Geometry: final body of the model. Coordinates: model frame, mm. Give positions to 0.01 mm unless a question says otherwise; leave off trailing zeros. Order: outer loops, then holes, each group sorted by start corner. A loop starts at its lowest first (then second) coordinate and runs counter-clockwise, first axis right, second up. Notation, with made-up numbers: (22, -33.5) -> (26, -33.5) arc R27 ccw to (26, -12.5) -> close; hole circle Ø3 at (56.5, 51.25). An arc over 180 degrees is marked (long way). Write item = value, one per line.
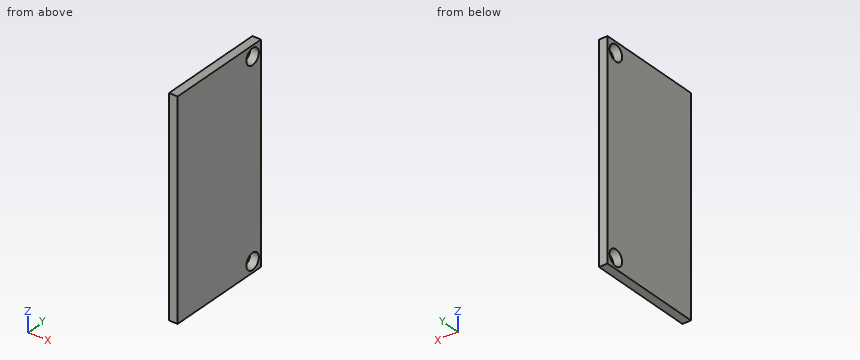
```python
from build123d import *

# Parameters (mm, degrees)
ESQUISSE1_W      = 40
ESQUISSE1_H      = 20
ESQUISSE1_R      = 1.5
EXTRUSION1_DEPTH = 1.6


with BuildPart() as part:
    # Esquisse1 → Extrusion1 (new body)
    with BuildSketch(Plane(origin=(0, 0, 0), x_dir=(0, 0, -1), z_dir=(1, 0, 0))):
        with Locations((0, 10)):
            Rectangle(ESQUISSE1_W, ESQUISSE1_H)
        with Locations((-18, 18)):
            Circle(ESQUISSE1_R, mode=Mode.SUBTRACT)
        with Locations(Location((18, 18, 0), (0, 0, 180))):
            Circle(ESQUISSE1_R, mode=Mode.SUBTRACT)
    extrude(amount=EXTRUSION1_DEPTH)


solid = part.part
```
1) First-contact query: P1, Ø4, axis at y = 10, z = 12.5, coming from the -X side; P2, Ø2.5, axis at y = 18, z = 18, coming from the +X side. Flat tips, straight axial feed; report the tip coordinate or a pass-through.
Check sheet entries:
P1 = 0
P2 = through
2) Section query C-C (x = 1). Output: boundary loops of the cut face in (y, z).
Check sheet entries:
outline = (0, -20) -> (20, -20) -> (20, 20) -> (0, 20) -> close; hole circle Ø3 at (18, -18); hole circle Ø3 at (18, 18)
3) Section query B-B (y = 18). Output: boundary loops of the cut face in (x, z), plus the area to 3 significant figures.
Check sheet entries:
outline = (0, -20) -> (1.6, -20) -> (1.6, -19.5) -> (0, -19.5) -> close; (0, -16.5) -> (1.6, -16.5) -> (1.6, 16.5) -> (0, 16.5) -> close; (0, 19.5) -> (1.6, 19.5) -> (1.6, 20) -> (0, 20) -> close
area = 54.4 mm²
4) Line query: line 1 (Y direction, x = 1.1, z = -18); line 2 (Y direction, x = 1.35, z = 17). Output: solid intervals per line, ascending. Write a range as from..to.
Check sheet entries:
line_1 = 0..16.5, 19.5..20
line_2 = 0..16.88, 19.12..20
5) Section query D-D (z = -17). Output: boundary loops of the cut face in (x, y).
Check sheet entries:
outline = (0, 0) -> (1.6, 0) -> (1.6, 16.88) -> (0, 16.88) -> close; (0, 19.12) -> (1.6, 19.12) -> (1.6, 20) -> (0, 20) -> close
6) Section query A-A (z = 18). Output: boundary loops of the cut face in (x, y).
Check sheet entries:
outline = (0, 0) -> (1.6, 0) -> (1.6, 16.5) -> (0, 16.5) -> close; (0, 19.5) -> (1.6, 19.5) -> (1.6, 20) -> (0, 20) -> close
